Can you work these out from the model? Positions are in its coordinate system, mm. Give positions to 0.01 mm unless a question says otherwise; leave off trailing zeros. Loops run counter-clockwise (first coordinate to the right, second up) from the corner with the lowest first, then second, coordinate; pieces in that order, holes last. Notation, with made-up numbers: (35.25, -20.5) - (82.25, -20.5) arc R29 ccw to (82.25, 5.5) - close; hole circle Ø8 at (65.25, 32). An arc over 180 degrees is marked (long way). Answer as a JSON object with one key per item and string values. Group by question number.
Item 1: Will these pins go through, and if not, where does the flat tip stop? pin 1 (1.5 mm diameter, centred on y = 5, z = 4.5, fed in from +X); pin 2 (1 mm diameter, centred on y = 2.5, z = 3, fed in from -X); pin 3 (1.5 mm diameter, centred on x = -3.5, z = 0.5, fed in from -Y); pin 4 (3 mm diameter, centred on x = 0, y = 0, fed in from +Z).
Item 2: Please list where these lines run through material, in increasing order: L1, parallel to Y at x = 0, z = 1.25; L2, parallel to Y at x = -0.75, z = 3.6; L3, parallel to X at y = -1.5, z = 2.15.
Item 3: Suppose I cut it at A-A on y = 0. Write out the boundary of the cut face in (x, z), and give its area (3 significant figures).
Item 4: Thinking about a two-plate mould opening in X: for faces 1 (the cylindrical face through (-5.158, 3.955, 2.472)), 2 (the flat face through (3, 0, 5)), 3 (the cylindrical face through (0, 2, 2)), which applies, pulls with the +X half, pulls with the -X half, needs draft (parallel to the pull), parting line crosses it, or undercut?
Item 5: Suppose I cut it at C-C on z = 4.2. Write out the boundary of the cut face in (x, y).
Autodesk Inventor part; units mm, degrees
ref_plane "YZ Plane" through (0, 0, 0) normal (1, 0, 0) x (0, 1, 0)
ref_plane "XZ Plane" through (0, 0, 0) normal (0, 1, 0) x (-1, 0, 0)
ref_plane "XY Plane" through (0, 0, 0) normal (0, 0, 1) x (1, 0, 0)
sketch "Sketch1" plane through (0, 0, 0) normal (0, 0, 1) x (1, 0, 0)
  circle A0 centre (0, 0) radius 6.5
  circle A1 centre (0, 0) radius 2
  dimension "d0" = 13
  dimension "d1" = 4
extrude "Extrusion1" add sketch "Sketch1" along normal blind 5
chamfer "Chamfer1" distance 0.5 angle 45 1 edges at (-6.5, 0, 5)
chamfer "Chamfer2" distance 0.5 angle 45 1 edges at (-6.5, 0, 0)
properties part number "4mmBearing"
Worked out:
{
 "1": {"pin 1": "stops at x = 4.92", "pin 2": "stops at x = -6.18", "pin 3": "stops at y = -5.89", "pin 4": "passes through"},
 "2": {"L1": "y = -6.5 to -2, 2 to 6.5", "L2": "y = -6.46 to -1.85, 1.85 to 6.46", "L3": "x = -6.32 to -1.32, 1.32 to 6.32"},
 "3": {"outline": "(-6.5, 0.5) - (-6, 0) - (-2, 0) - (-2, 5) - (-6, 5) - (-6.5, 4.5) - close; (2, 0) - (6, 0) - (6.5, 0.5) - (6.5, 4.5) - (6, 5) - (2, 5) - close", "area": "44.5 mm2"},
 "4": {"face 1": "parting line crosses it", "face 2": "needs draft", "face 3": "undercut"},
 "5": {"outline": "circle Ø13 at (0, 0); hole circle Ø4 at (0, 0)"}
}
